Input: part model. Units: mm. Frame: model coordinates. Face numbers are marked on the shaded views. Coordinates: 2 decimals unless noted, no trailing zeros. Write each loop counter-clockwise with the first axis right and the second up, starting at its lowest first coordinate (ties: lowest second). Pieces come first, ordered by that corner, then holes.
1) Pin query (flat end, axial travel): pin 1 Ø1 at (x, z) = (6621.5, 1261) entering from -Y; pin 2 Ø20.5 at (x, y) = (5923, 2622) entering from -Z. Return the tip coordinate at first contact, or that it passes through.
2) Section query A-A (z = 1754). Output: boundary loops of the cut face in (x, y), then the cut area to 3 significant figures.
3) Section query B-B (x = 6697.5). Output: boundary loops of the cut face in (y, z), then the cut area to 3 significant figures.
4) Draft query along Z for the marked faces 1, 2 and 3. Return one class per face: pulls with the +Z half, pulls with the -Z half, needs draft (parallel to the pull), parting line crosses it, or undercut.
5) Line query: L1, parallel to Y at x = 6513, z = 249. Output: solid intervals per line, ascending.
from build123d import *

# Parameters (mm, degrees)
BOX017_W     = 1168.4
BOX017_H     = 25.4
BOX017_DEPTH = 2082.8
BOX016_W     = 1219.2
BOX016_H     = 609.6
BOX016_DEPTH = 2133.6


with BuildPart() as cube017:
    # Box017 → Box017 (new body)
    with BuildSketch(Plane(origin=(25.4, 0, 25.4), x_dir=(1, 0, 0), z_dir=(0, 0, 1))):
        with Locations((584.2, 12.7)):
            Rectangle(BOX017_W, BOX017_H)
    extrude(amount=BOX017_DEPTH)


with BuildPart() as cut005:
    # Box016 → Box016 (new body)
    with BuildSketch(Plane.XY):
        with Locations((609.6, 304.8)):
            Rectangle(BOX016_W, BOX016_H)
    extrude(amount=BOX016_DEPTH)

    # Cut005: cut Cube017
    add(cube017.part, mode=Mode.SUBTRACT)


with BuildPart() as cut005_1:
    # Cut005 placement: moved
    add(cut005.part.moved(Location((5575, 2613, 0))))


solid = cut005_1.part
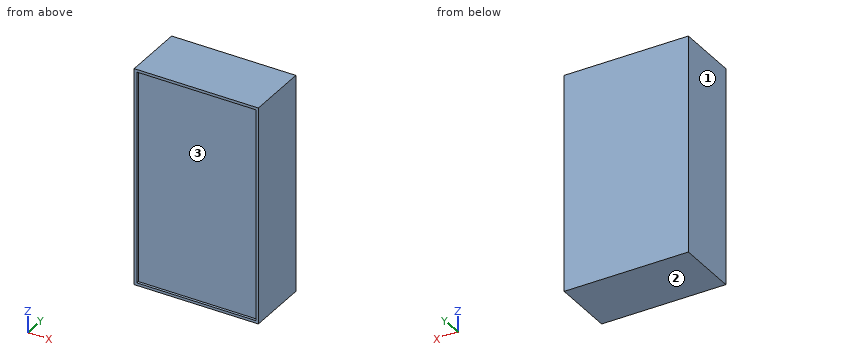
Answer:
1. pin 1: stops at y = 2638.4
1. pin 2: stops at z = 0
2. outline: (5575, 2613) - (5600.4, 2613) - (5600.4, 2638.4) - (6768.8, 2638.4) - (6768.8, 2613) - (6794.2, 2613) - (6794.2, 3222.6) - (5575, 3222.6) - close
2. area: 714,000 mm2
3. outline: (2613, 0) - (3222.6, 0) - (3222.6, 2133.6) - (2613, 2133.6) - (2613, 2108.2) - (2638.4, 2108.2) - (2638.4, 25.4) - (2613, 25.4) - close
3. area: 1,250,000 mm2
4. face 1: needs draft
4. face 2: pulls with the -Z half
4. face 3: undercut
5. L1: y = 2638.4 to 3222.6
